```python
from build123d import *

# Parameters (mm, degrees)
SKETCH1_W           = 55
SKETCH1_H           = 50
BOSS_EXTRUDE1_DEPTH = 10.7
SKETCH2_W           = 30.6
SKETCH2_H           = 40.3
CUT_EXTRUDE2_DEPTH  = 3
SKETCH4_W           = 40.6
SKETCH4_H           = 40.3
CUT_EXTRUDE3_DEPTH  = 3.2
SKETCH13_R          = 3
CUT_EXTRUDE4_DEPTH  = 2.5
SKETCH14_R          = 1
CUT_EXTRUDE5_DEPTH  = 2


with BuildPart() as part:
    # Sketch1 → Boss-Extrude1 (new body)
    with BuildSketch(Plane(origin=(0, 0, 0), x_dir=(1, 0, 0), z_dir=(0, 1, 0))):
        Rectangle(SKETCH1_W, SKETCH1_H)
    extrude(amount=BOSS_EXTRUDE1_DEPTH)

    # Sketch2 → Cut-Extrude2 (cut)
    with BuildSketch(Plane(origin=(0, 10.7, 0), x_dir=(1, 0, 0), z_dir=(0, 1, 0))):
        with Locations((0, 4.85)):
            Rectangle(SKETCH2_W, SKETCH2_H)
    extrude(amount=-CUT_EXTRUDE2_DEPTH, mode=Mode.SUBTRACT)

    # Sketch4 → Cut-Extrude3 (cut)
    with BuildSketch(Plane(origin=(0, 7.7, 0), x_dir=(1, 0, 0), z_dir=(0, 1, 0))):
        with Locations((0, 4.85)):
            Rectangle(SKETCH4_W, SKETCH4_H)
    extrude(amount=-CUT_EXTRUDE3_DEPTH, mode=Mode.SUBTRACT)

    # Sketch13 → Cut-Extrude4 (cut)
    with BuildSketch(Plane(origin=(0, 4.5, 0), x_dir=(1, 0, 0), z_dir=(0, 1, 0))):
        with Locations(Location((0, 12.850318005, 0), (0, 0, 270))):
            Circle(SKETCH13_R)
        with Locations(Location((0, -2.359937211, 0), (0, 0, 270))):
            Circle(SKETCH13_R)
    extrude(amount=-CUT_EXTRUDE4_DEPTH, mode=Mode.SUBTRACT)

    # Sketch14 → Cut-Extrude5 (cut)
    with BuildSketch(Plane(origin=(0, 2, 0), x_dir=(1, 0, 0), z_dir=(0, 1, 0))):
        with Locations(Location((0, 12.850318005, 0), (0, 0, 270))):
            Circle(SKETCH14_R)
        with Locations(Location((0, -2.149681995, 0), (0, 0, 270))):
            Circle(SKETCH14_R)
    extrude(amount=-CUT_EXTRUDE5_DEPTH, mode=Mode.SUBTRACT)


solid = part.part
```
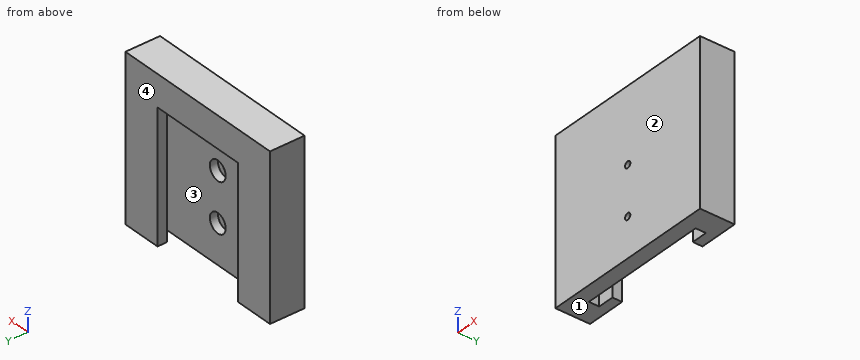
Check sheet for the modelled part. Datum: model origin and axes. Units: mm. Face numbers are marked on the shaded views. Give positions to 0.01 mm unless a question says otherwise; leave off trailing zeros. Write each loop counter-clockwise with the first axis right and the second up, starting at its lowest first coordinate (ties: lowest second). Pieces come first, ordered by that corner, then holes.
Item 1: Cross-section at B-B (x = -18). Enter the section's corners in (y, z).
Item 2: Scan lines: L1, parallel to Y at x = 20, z = -10.5; L2, parallel to X at y = 5, z = 2.5; L3, parallel to X at y = 8.25, z = -1.5. Record each from-to range of solid material in increasing order.
Item 3: Cross-section at C-C (x = 0). Enter the section's corners in (y, z), and give its area (3 significant figures).
Item 4: Draft check along Y on the marked faces 1, 2, 3 and 4. Enter one of: released by +Y, released by -Y, zero draft, split by the parting line, or undercut.
Item 5: Gauge pin test, flat ends, axial feed: pin 1 (1.8 mm diameter, centred on x = 1, z = 3.5, fed in from +Y); pin 2 (5 mm diameter, centred on x = 0.5, z = -14.5, fed in from +Y). Record the tip position at first contact, or that the pin passes through.
Item 6: Cross-section at D-D (z = -17). Enter the section's corners in (x, y), and give its area (3 significant figures).
Item 7: Cross-section at A-A (y = 8.75). Enter the section's corners in (x, z), and give its area (3 significant figures).
Report:
1. outline: (0, -25) - (4.5, -25) - (4.5, 15.3) - (7.7, 15.3) - (7.7, -25) - (10.7, -25) - (10.7, 25) - (0, 25) - close
2. L1: y = 0 to 4.5, 7.7 to 10.7
2. L2: x = -27.5 to -20.3, 20.3 to 27.5
2. L3: x = -27.5 to -15.3, 15.3 to 27.5
3. outline: (0, -25) - (4.5, -25) - (4.5, -15.85) - (2, -15.85) - (2, -13.85) - (0, -13.85) - close; (0, -11.85) - (2, -11.85) - (2, -9.85) - (4.5, -9.85) - (4.5, -0.64) - (2, -0.64) - (2, 1.15) - (0, 1.15) - close; (0, 3.15) - (2, 3.15) - (2, 5.36) - (4.5, 5.36) - (4.5, 15.3) - (10.7, 15.3) - (10.7, 25) - (0, 25) - close
3. area: 247 mm2
4. face 1: zero draft
4. face 2: released by -Y
4. face 3: undercut
4. face 4: released by +Y
5. pin 1: stops at y = 2
5. pin 2: stops at y = 4.5
6. outline: (-27.5, 0) - (27.5, 0) - (27.5, 10.7) - (15.3, 10.7) - (15.3, 7.7) - (20.3, 7.7) - (20.3, 4.5) - (-20.3, 4.5) - (-20.3, 7.7) - (-15.3, 7.7) - (-15.3, 10.7) - (-27.5, 10.7) - close
6. area: 367 mm2
7. outline: (-27.5, -25) - (-15.3, -25) - (-15.3, 15.3) - (15.3, 15.3) - (15.3, -25) - (27.5, -25) - (27.5, 25) - (-27.5, 25) - close
7. area: 1,520 mm2
